from build123d import *

# Parameters (mm, degrees)
SKETCH_1_W          = 200
SKETCH_1_H          = 245
EXTRUDE_1_DEPTH     = 20
CUT_EXTRUDE_1_REACH = 161.393
SKETCH_2_R          = 7
CHAMFER_1_SIZE      = 5


with BuildPart() as part:
    # 草图1 → 凸台-拉伸1 (new body)
    with BuildSketch(Plane.XY):
        Rectangle(SKETCH_1_W, SKETCH_1_H)
    extrude(amount=EXTRUDE_1_DEPTH)

    # 草图2 → 切除-拉伸1 (cut, up to next)
    with BuildSketch(Plane.XY.offset(20), mode=Mode.PRIVATE) as cut_extrude_1_sk1:
        with Locations((-54, 60)):
            Circle(SKETCH_2_R)
    cut_extrude_1_tool1 = extrude(cut_extrude_1_sk1.sketch, amount=-CUT_EXTRUDE_1_REACH, mode=Mode.PRIVATE) & part.part
    # 草图2 → 切除-拉伸1 (cut, up to next)
    with BuildSketch(Plane.XY.offset(20), mode=Mode.PRIVATE) as cut_extrude_1_sk2:
        with Locations((0, 60)):
            Circle(SKETCH_2_R)
    cut_extrude_1_tool2 = extrude(cut_extrude_1_sk2.sketch, amount=-CUT_EXTRUDE_1_REACH, mode=Mode.PRIVATE) & part.part
    # 草图2 → 切除-拉伸1 (cut, up to next)
    with BuildSketch(Plane.XY.offset(20), mode=Mode.PRIVATE) as cut_extrude_1_sk3:
        with Locations((54, 60)):
            Circle(SKETCH_2_R)
    cut_extrude_1_tool3 = extrude(cut_extrude_1_sk3.sketch, amount=-CUT_EXTRUDE_1_REACH, mode=Mode.PRIVATE) & part.part
    # 草图2 → 切除-拉伸1 (cut, up to next)
    with BuildSketch(Plane.XY.offset(20), mode=Mode.PRIVATE) as cut_extrude_1_sk4:
        with Locations((-54, 0)):
            Circle(SKETCH_2_R)
    cut_extrude_1_tool4 = extrude(cut_extrude_1_sk4.sketch, amount=-CUT_EXTRUDE_1_REACH, mode=Mode.PRIVATE) & part.part
    # 草图2 → 切除-拉伸1 (cut, up to next)
    with BuildSketch(Plane.XY.offset(20), mode=Mode.PRIVATE) as cut_extrude_1_sk5:
        with Locations((54, 0)):
            Circle(SKETCH_2_R)
    cut_extrude_1_tool5 = extrude(cut_extrude_1_sk5.sketch, amount=-CUT_EXTRUDE_1_REACH, mode=Mode.PRIVATE) & part.part
    # 草图2 → 切除-拉伸1 (cut, up to next)
    with BuildSketch(Plane.XY.offset(20), mode=Mode.PRIVATE) as cut_extrude_1_sk6:
        with Locations((-54, -60)):
            Circle(SKETCH_2_R)
    cut_extrude_1_tool6 = extrude(cut_extrude_1_sk6.sketch, amount=-CUT_EXTRUDE_1_REACH, mode=Mode.PRIVATE) & part.part
    # 草图2 → 切除-拉伸1 (cut, up to next)
    with BuildSketch(Plane.XY.offset(20), mode=Mode.PRIVATE) as cut_extrude_1_sk7:
        with Locations((0, -60)):
            Circle(SKETCH_2_R)
    cut_extrude_1_tool7 = extrude(cut_extrude_1_sk7.sketch, amount=-CUT_EXTRUDE_1_REACH, mode=Mode.PRIVATE) & part.part
    # 草图2 → 切除-拉伸1 (cut, up to next)
    with BuildSketch(Plane.XY.offset(20), mode=Mode.PRIVATE) as cut_extrude_1_sk8:
        with Locations((54, -60)):
            Circle(SKETCH_2_R)
    cut_extrude_1_tool8 = extrude(cut_extrude_1_sk8.sketch, amount=-CUT_EXTRUDE_1_REACH, mode=Mode.PRIVATE) & part.part
    # 草图2 → 切除-拉伸1 (cut, up to next)
    with BuildSketch(Plane.XY.offset(20), mode=Mode.PRIVATE) as cut_extrude_1_sk9:
        with BuildLine():
            Line((-31, 47), (31, 47))
            ThreePointArc((31, 47), (38.071067812, 44.071067812), (41, 37))
            Line((41, 37), (41, -37))
            ThreePointArc((41, -37), (38.071067812, -44.071067812), (31, -47))
            Line((31, -47), (-31, -47))
            ThreePointArc((-31, -47), (-38.071067812, -44.071067812), (-41, -37))
            Line((-41, -37), (-41, 37))
            ThreePointArc((-41, 37), (-38.071067812, 44.071067812), (-31, 47))
        make_face()
    cut_extrude_1_tool9 = extrude(cut_extrude_1_sk9.sketch, amount=-CUT_EXTRUDE_1_REACH, mode=Mode.PRIVATE) & part.part
    add(cut_extrude_1_tool1.solids().sort_by_distance((-54, 60, 20))[0], mode=Mode.SUBTRACT)
    add(cut_extrude_1_tool2.solids().sort_by_distance((0, 60, 20))[0], mode=Mode.SUBTRACT)
    add(cut_extrude_1_tool3.solids().sort_by_distance((54, 60, 20))[0], mode=Mode.SUBTRACT)
    add(cut_extrude_1_tool4.solids().sort_by_distance((-54, 0, 20))[0], mode=Mode.SUBTRACT)
    add(cut_extrude_1_tool5.solids().sort_by_distance((54, 0, 20))[0], mode=Mode.SUBTRACT)
    add(cut_extrude_1_tool6.solids().sort_by_distance((-54, -60, 20))[0], mode=Mode.SUBTRACT)
    add(cut_extrude_1_tool7.solids().sort_by_distance((0, -60, 20))[0], mode=Mode.SUBTRACT)
    add(cut_extrude_1_tool8.solids().sort_by_distance((54, -60, 20))[0], mode=Mode.SUBTRACT)
    add(cut_extrude_1_tool9.solids().sort_by_distance((0, 0, 20))[0], mode=Mode.SUBTRACT)

    # 倒角1
    chamfer_1_edges = [part.edges().sort_by_distance(p)[0] for p in [
        (0, -122.5, 0),
        (0, 122.5, 0),
    ]]
    chamfer(chamfer_1_edges, length=CHAMFER_1_SIZE)


solid = part.part
Geometry check sheet. Reference: the model listing, model coordinates, mm. A direction names the side the tool comes from. Round coordinates to 2 decimals unless told otherwise and drop trailing zeros. Order: outer loops, then holes, each group sorted by start corner. A loop starts at its lowest first (then second) coordinate and runs counter-clockwise, first axis right, second up. Notation, with made-up numbers: M 6.25,-11.75 L 20.25,-11.75 A9 ccw 20.25,-7.75 Z; hole C -38.5,33.25 d2. An arc over 180 degrees is marked long. Write each question's results on one line, items separated by ' | '. Start each with the question number.
1. Set-up check for faces 4 (the face through (-1.4, -120, 2.5)), 5 (the face through (-41, -1, 10)): record each of +Z, -Z, +X, -X, +Y, -Y from which the full face is reachable in a straight line by a thin tool's end or side.
2. Cross-section at A-A on x = 28. Record the boundary of the cut face in (y, z).
3. Draft check along Y on faces 1 (the face through (-100, -2, 10)), 2 (the face through (-0.91, -53.06, 10.14)), 3 (the face through (-1, 122.5, 12)). Enter one of: pulls with the +Y half, pulls with the -Y half, needs draft (parallel to the pull), parting line crosses it, or undercut.
4. Material ranges on L1, parallel to Y at x = 54, z = 14; L2, parallel to X at y = -31, z = 9; L3, parallel to Y at x = 18.5, z = 7, recorded low to high. Write a range as from..to.
5. Cross-section at B-B on y = -60. Record the boundary of the cut face in (x, z).
6. Cross-section at D-D on y = -16. Record the boundary of the cut face in (x, z).
7. Cross-section at C-C on z = 10.75. Give the number of separate pieces and of enclosed holes in the cut face, plus the area to 3 significant figures.
8. Go/stop test with flat-tipped pins: P1, Ø8.5, axis at x = -54, y = -60, coming from the +Z side; P2, Ø1.5, axis at x = 69, z = 2, coming from the -Y side. Record where each tip stops, or that it passes through.
Resolved:
1) face 4: -Z, +X, -X, -Y | face 5: +Z, -Z
2) outline: M -122.5,5 L -117.5,0 L -47,0 L -47,20 L -122.5,20 Z; M 47,0 L 117.5,0 L 122.5,5 L 122.5,20 L 47,20 Z
3) face 1: needs draft | face 2: undercut | face 3: pulls with the +Y half
4) L1: -122.5..-67, -53..-7, 7..53, 67..122.5 | L2: -100..-41, 41..100 | L3: -122.5..-47, 47..122.5
5) outline: M -100,0 L -61,0 L -61,20 L -100,20 Z; M -47,0 L -7,0 L -7,20 L -47,20 Z; M 7,0 L 47,0 L 47,20 L 7,20 Z; M 61,0 L 100,0 L 100,20 L 61,20 Z
6) outline: M -100,0 L -41,0 L -41,20 L -100,20 Z; M 41,0 L 100,0 L 100,20 L 41,20 Z
7) separate pieces: 1 | enclosed holes: 9 | area: 40,100 mm2
8) P1: through | P2: y = -120.25
